Design review of the part built by this model. Coordinates are the model's own, in mm. A direction names the side the tool comes from. Give positions to 0.01 mm unless a question says otherwise; leave off trailing zeros. Write each loop counter-clockwise with the first axis right and the second up, starting at its lowest first coordinate (ties: lowest second). Pieces come first, ordered by that corner, then holes. Notation, with made-up numbers: (89, 13) - (95, 13) arc R8 ccw to (95, 19) - close; hole circle Ø3 at (-12, -34.5). An arc over 180 degrees is marked (long way). Use a Markdown table: item, result. Add a question column.
```python
from build123d import *

# Parameters (mm, degrees)
BOSS_EXTRUDE1_DEPTH = 1219.2
FILLET1_R           = 0.254
SKETCH4_W           = 1905.2
SKETCH4_H           = 92.573708452
CUT_EXTRUDE1_DEPTH  = 60
SKETCH9_R           = 1.65
CUT_EXTRUDE6_DEPTH  = 60
SKETCH10_R          = 1.65
CUT_EXTRUDE7_DEPTH  = 60


with BuildPart() as part:
    # Sketch3 → Boss-Extrude1 (new, symmetric)
    with BuildSketch(Plane.XY):
        Polygon((1.5875, 25.4), (0, 25.4), (0, 0), (25.4, 0), (25.4, 1.5875), (1.5875, 1.5875), align=None)
    extrude(amount=BOSS_EXTRUDE1_DEPTH, both=True)

    # Fillet1
    fillet1_edges = [part.edges().sort_by_distance(p)[0] for p in [
        (1.5875, 1.5875, 0),
    ]]
    fillet(fillet1_edges, radius=FILLET1_R)

    # Sketch4 → Cut-Extrude1 (cut)
    with BuildSketch(Plane.ZY):
        with Locations((-266.6, -7.427787689)):
            Rectangle(SKETCH4_W, SKETCH4_H)
    extrude(amount=-CUT_EXTRUDE1_DEPTH, mode=Mode.SUBTRACT)

    # Sketch9 → Cut-Extrude6 (cut)
    with BuildSketch(Plane(origin=(0, 1.5875, 0), x_dir=(1, 0, 0), z_dir=(0, 1, 0))):
        with Locations(Location((11.113, -1208.791795667, 0), (0, 0, 180))):
            Circle(SKETCH9_R)
        with Locations(Location((11.1125, -696.408204333, 0), (0, 0, 180))):
            Circle(SKETCH9_R)
        with Locations(Location((13.49375, -1182.6, 0), (0, 0, 180))):
            Circle(SKETCH9_R)
        with Locations(Location((13.49375, -1162.6, 0), (0, 0, 180))):
            Circle(SKETCH9_R)
        with Locations(Location((13.49375, -1142.6, 0), (0, 0, 180))):
            Circle(SKETCH9_R)
        with Locations(Location((13.49375, -1122.6, 0), (0, 0, 180))):
            Circle(SKETCH9_R)
        with Locations(Location((13.49375, -1102.6, 0), (0, 0, 180))):
            Circle(SKETCH9_R)
        with Locations(Location((13.49375, -1082.6, 0), (0, 0, 180))):
            Circle(SKETCH9_R)
        with Locations(Location((13.49375, -1062.6, 0), (0, 0, 180))):
            Circle(SKETCH9_R)
        with Locations(Location((13.49375, -1042.6, 0), (0, 0, 180))):
            Circle(SKETCH9_R)
        with Locations(Location((13.49375, -1022.6, 0), (0, 0, 180))):
            Circle(SKETCH9_R)
        with Locations(Location((13.49375, -1002.6, 0), (0, 0, 180))):
            Circle(SKETCH9_R)
        with Locations(Location((13.49375, -982.6, 0), (0, 0, 180))):
            Circle(SKETCH9_R)
        with Locations(Location((13.49375, -962.6, 0), (0, 0, 180))):
            Circle(SKETCH9_R)
        with Locations(Location((13.49375, -942.6, 0), (0, 0, 180))):
            Circle(SKETCH9_R)
        with Locations(Location((13.49375, -922.6, 0), (0, 0, 180))):
            Circle(SKETCH9_R)
        with Locations(Location((13.49375, -902.6, 0), (0, 0, 180))):
            Circle(SKETCH9_R)
        with Locations(Location((13.49375, -882.6, 0), (0, 0, 180))):
            Circle(SKETCH9_R)
        with Locations(Location((13.49375, -862.6, 0), (0, 0, 180))):
            Circle(SKETCH9_R)
        with Locations(Location((13.49375, -842.6, 0), (0, 0, 180))):
            Circle(SKETCH9_R)
        with Locations(Location((13.49375, -822.6, 0), (0, 0, 180))):
            Circle(SKETCH9_R)
        with Locations(Location((13.49375, -802.6, 0), (0, 0, 180))):
            Circle(SKETCH9_R)
        with Locations(Location((13.49375, -782.6, 0), (0, 0, 180))):
            Circle(SKETCH9_R)
        with Locations(Location((13.49375, -762.6, 0), (0, 0, 180))):
            Circle(SKETCH9_R)
        with Locations(Location((13.49375, -742.6, 0), (0, 0, 180))):
            Circle(SKETCH9_R)
        with Locations(Location((13.49375, -722.6, 0), (0, 0, 180))):
            Circle(SKETCH9_R)
    extrude(amount=-CUT_EXTRUDE6_DEPTH, mode=Mode.SUBTRACT)

    # Sketch10 → Cut-Extrude7 (cut)
    with BuildSketch(Plane(origin=(1.5875, 0, 0), x_dir=(0, 0, -1), z_dir=(1, 0, 0))):
        with Locations((-703.4625, 10.3759)):
            Circle(SKETCH10_R)
        with Locations((-1201.7375, 10.3759)):
            Circle(SKETCH10_R)
        with Locations((-728.1, 13.49375)):
            Circle(SKETCH10_R)
        with Locations((-771.1, 13.49375)):
            Circle(SKETCH10_R)
        with Locations((-814.1, 13.49375)):
            Circle(SKETCH10_R)
        with Locations((-857.1, 13.49375)):
            Circle(SKETCH10_R)
        with Locations((-877.1, 13.49375)):
            Circle(SKETCH10_R)
        with Locations((-897.1, 13.49375)):
            Circle(SKETCH10_R)
        with Locations((-917.1, 13.49375)):
            Circle(SKETCH10_R)
        with Locations((-937.1, 13.49375)):
            Circle(SKETCH10_R)
        with Locations((-957.1, 13.49375)):
            Circle(SKETCH10_R)
        with Locations((-977.1, 13.49375)):
            Circle(SKETCH10_R)
        with Locations((-997.1, 13.49375)):
            Circle(SKETCH10_R)
        with Locations((-1017.1, 13.49375)):
            Circle(SKETCH10_R)
        with Locations((-1037.1, 13.49375)):
            Circle(SKETCH10_R)
        with Locations((-1057.1, 13.49375)):
            Circle(SKETCH10_R)
        with Locations((-1077.1, 13.49375)):
            Circle(SKETCH10_R)
        with Locations((-1097.1, 13.49375)):
            Circle(SKETCH10_R)
        with Locations((-1117.1, 13.49375)):
            Circle(SKETCH10_R)
        with Locations((-1137.1, 13.49375)):
            Circle(SKETCH10_R)
        with Locations((-1157.1, 13.49375)):
            Circle(SKETCH10_R)
        with Locations((-1177.1, 13.49375)):
            Circle(SKETCH10_R)
    extrude(amount=-CUT_EXTRUDE7_DEPTH, mode=Mode.SUBTRACT)


solid = part.part
```
(1) Insertion check: pin 1 (5.5 mm diameter, centred on x = 13.49, z = 902.6, fed in from +Y); pin 2 (4.5 mm diameter, centred on x = 13.49, z = 1162.6, fed in from -Y); pin 3 (10 mm diameter, centred on y = 16, z = 1103.5, fed in from +X). Each pin has a flat end and moves straight along its axis. Give the tip position at first contact, or say it passes through.
(2) Add section B-B (y = 19.75). State the section outline as (x, z) points.
(3) Tool access review of faces 1 (the face through (1, 7, 1219.2)), 2 (the face through (1.588, 16, 956)): name each direction out of +Z, -Z, +X, -X, +Y, -Y from which nothing blocks a thin tool from reaching the whole face with its end or side.
(4) Add section A-A (z = 735). State the section outline as (x, y) points.
(5) For line 1 along X through (y, z) = (0.6, 942.6); line 2 along Y through (x, z) = (19.25, 1068), list the stretches that pass through material, from the lowest coordinate up.
Answers follow:
| question | item | result |
|---|---|---|
| 1 | pin 1 | y = 1.59 |
| 1 | pin 2 | y = 0 |
| 1 | pin 3 | x = 1.59 |
| 2 | outline | (0, 686) - (1.59, 686) - (1.59, 1219.2) - (0, 1219.2) - close |
| 3 | face 1 | +Z, +X, -X, +Y, -Y |
| 3 | face 2 | +Z, -Z, +X, +Y |
| 4 | outline | (0, 0) - (25.4, 0) - (25.4, 1.59) - (1.84, 1.59) arc R0.25 cw to (1.59, 1.84) - (1.59, 25.4) - (0, 25.4) - close |
| 5 | line 1 | 0 to 11.84, 15.14 to 25.4 |
| 5 | line 2 | 0 to 1.59 |
